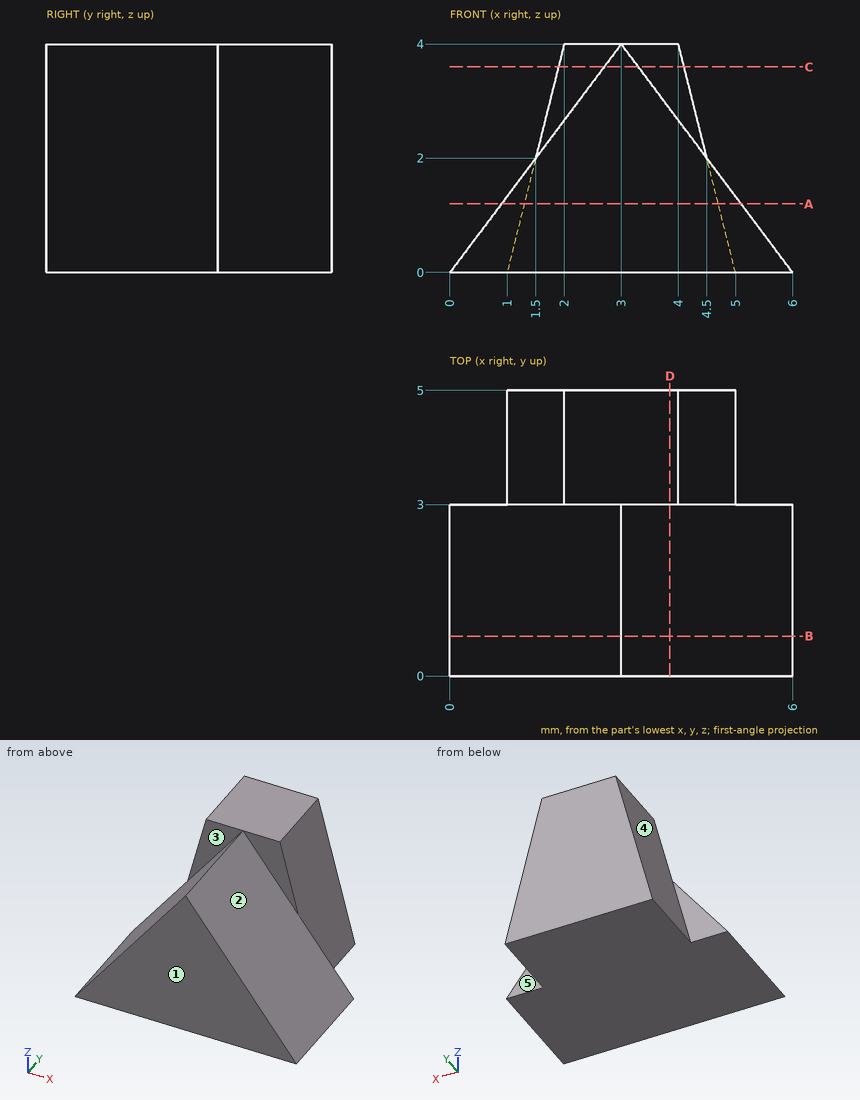
Geometry check sheet. Reference: drawing and pictorial views, mm from the part's lowest x, y, z. A direction names the side the tool comes from. Round coordinates to 2 decimals unless told otherwise and drop trailing zeros. Order: outer loops, then holes, each group sorted by start corner. A loop starts at its lowest first (then second) coordinate and runs counter-clockwise, first axis right, second up.
Q1. Scan lines: L1, parallel to Y at x = 5, z = 0.35; L2, parallel to X at y = 1.8, z = 1.6. Record each from-to range of solid material in increasing order.
Filled sheet:
L1: y = 0 to 3
L2: x = 1.2 to 4.8
Q2. Cross-section at B-B, the plane y = 0.7. Enter the section's corners in (x, z).
Filled sheet:
outline: (0, 0) - (6, 0) - (3, 4) - close
Q3. Set-up check for the marked faces 1, 2, 3, 4 and 5: record each of +Z, -Z, +X, -X, +Y, -Y from which the full face is reachable in a straight line by a thin tool's end or side.
Filled sheet:
face 1: +Z, -Z, +X, -X, -Y
face 2: +Z, +X, -Y
face 3: +Z, -X, -Y
face 4: +Z, -X, +Y
face 5: +Z, +X, +Y
Q4. Cross-section at C-C, the plane z = 3.6. Enter the section's corners in (x, y).
Filled sheet:
outline: (1.9, 3) - (2.7, 3) - (2.7, 0) - (3.3, 0) - (3.3, 3) - (4.1, 3) - (4.1, 5) - (1.9, 5) - close
Q5. Cross-section at D-D, the plane x = 3.85. Enter the section's corners in (y, z), plus the area to 3 significant figures.
Filled sheet:
outline: (0, 0) - (5, 0) - (5, 4) - (3, 4) - (3, 2.87) - (0, 2.87) - close
area: 16.6 mm2
Q6. Cross-section at A-A, the plane z = 1.2. Enter the section's corners in (x, y), plus the area to 3 significant figures.
Filled sheet:
outline: (0.9, 0) - (5.1, 0) - (5.1, 3) - (4.7, 3) - (4.7, 5) - (1.3, 5) - (1.3, 3) - (0.9, 3) - close
area: 19.4 mm2
Q7. Depth check by flat-ended pin: P1, Ø2, axis at y = 1.5, z = 3, coming from the -X side; P2, Ø1.5, axis at y = 4, z = 0.5, coming from the +X side; P3, Ø0.8, axis at x = 0.5, z = 0.5, coming from the +Y side. Enter the tip coordinate at first touch or a pass-through.
Filled sheet:
P1: stops at x = 1.5
P2: stops at x = 5
P3: stops at y = 3
